```python
from build123d import *

# Parameters (mm, degrees)
SKETCH1_R           = 25.25
SKETCH1_R_2         = 4.25
BOSS_EXTRUDE1_DEPTH = 10
SHELL1_T            = -2
SKETCH2_R           = 63.400619105
CUT_EXTRUDE1_DEPTH  = 29


with BuildPart() as part:
    # Sketch1 → Boss-Extrude1 (new body)
    with BuildSketch(Plane.YZ):
        with BuildLine():
            Line((-50, 72), (50, 72))
            ThreePointArc((50, 72), (65.556349186, 65.556349186), (72, 50))
            Line((72, 50), (72, -50))
            ThreePointArc((72, -50), (65.556349186, -65.556349186), (50, -72))
            Line((50, -72), (-50, -72))
            ThreePointArc((-50, -72), (-65.556349186, -65.556349186), (-72, -50))
            Line((-72, -50), (-72, 50))
            ThreePointArc((-72, 50), (-65.556349186, 65.556349186), (-50, 72))
        make_face()
        with Locations(Location((34, 0, 0), (0, 0, 270))):
            Circle(SKETCH1_R, mode=Mode.SUBTRACT)
        with Locations(Location((-34, -14.79, 0), (0, 0, 270))):
            Circle(SKETCH1_R_2, mode=Mode.SUBTRACT)
    extrude(amount=BOSS_EXTRUDE1_DEPTH)

    # Shell1
    shell1_openings = [part.faces().sort_by_distance(p)[0] for p in [
        (10, -3.623679056, 0.045959525),
    ]]
    offset(amount=SHELL1_T, openings=shell1_openings, kind=Kind.INTERSECTION)

    # Sketch2 → Cut-Extrude1 (cut)
    with BuildSketch(Plane.YZ.offset(2)):
        Circle(SKETCH2_R)
    extrude(amount=CUT_EXTRUDE1_DEPTH, mode=Mode.SUBTRACT)


solid = part.part
```
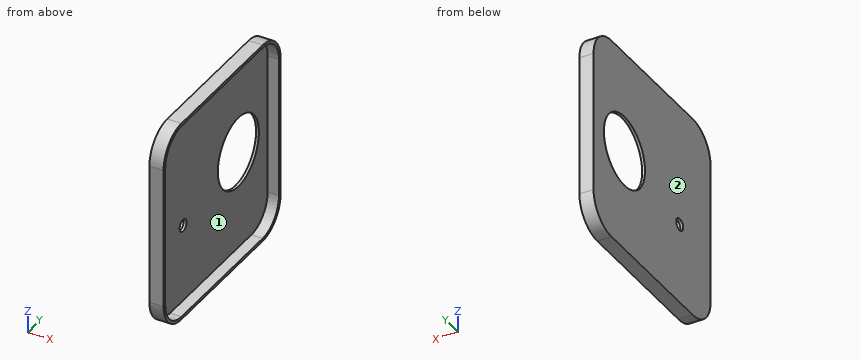
Could you check a few things on this model? Use its own coordinates, in mm. Face numbers are marked on the shaded views. Coordinates: 2 decimals unless noted, no trailing zeros. Loops run counter-clockwise (first coordinate to the right, second up) from the corner with the lowest first, then second, coordinate; pieces in that order, holes last.
1) Will this pin go through, and if not, where does the flat tip stop? pin 1 Ø6 at (y, z) = (18, 35.5) entering from +X.
Reported:
pin 1: stops at x = 2
2) Imagine slicing it at A-A (z = 0). List the corners of the cut face in (x, y) for me, and give its area (3 significant figures).
Reported:
outline: (0, -72) - (10, -72) - (10, -70) - (2, -70) - (2, 8.75) - (0, 8.75) - close; (0, 59.25) - (2, 59.25) - (2, 70) - (10, 70) - (10, 72) - (0, 72) - close
area: 219 mm2
3) Imagine slicing it at C-C (x = 5.75). List the corners of the cut face in (y, z) for me.
Reported:
outline: (-72, -50) arc R22 ccw to (-50, -72) - (50, -72) arc R22 ccw to (72, -50) - (72, 50) arc R22 ccw to (50, 72) - (-50, 72) arc R22 ccw to (-72, 50) - close; hole (-70, -50) arc R20 ccw to (-50, -70) - (50, -70) arc R20 ccw to (70, -50) - (70, 50) arc R20 ccw to (50, 70) - (-50, 70) arc R20 ccw to (-70, 50) - close
4) Imagine slicing it at B-B (y = -34). List the corners of the cut face in (x, z) for me, and give its area (3 significant figures).
Reported:
outline: (0, -72) - (10, -72) - (10, -70) - (2, -70) - (2, -19.04) - (0, -19.04) - close; (0, -10.54) - (2, -10.54) - (2, 70) - (10, 70) - (10, 72) - (0, 72) - close
area: 303 mm2
5) Thinking about a two-plate mould opening in Z: for the marked faces 1 and 2, which applies, released by +Z, released by -Z, zero draft, split by the parting line, or undercut?
Reported:
face 1: undercut
face 2: zero draft
6) Please list where these lines run through material, in increasing order: line 1 along Z through (x, y) = (0.9, 34); line 2 along Y through (x, z) = (7, -38).
Reported:
line 1: z = -72 to -25.25, 25.25 to 72
line 2: y = -72 to -70, 70 to 72
7) Imagine slicing it at D-D (z = -37.5). List the corners of the cut face in (x, y) for me, and give its area (3 significant figures).
Reported:
outline: (0, -72) - (10, -72) - (10, -70) - (2, -70) - (2, 70) - (10, 70) - (10, 72) - (0, 72) - close
area: 320 mm2
